```python
from build123d import *

# Parameters (mm, degrees)
SKETCH1_W            = 10
SKETCH1_H            = 80
BOSS_EXTRUDE1_DEPTH  = 51
SKETCH2_R            = 7.75
CUT_EXTRUDE1_DEPTH   = 45.1
SKETCH3_R            = 4.5
CUT_EXTRUDE2_DEPTH   = 96.399161422
SKETCH4_W            = 30
SKETCH4_H            = 80
SKETCH4_R            = 4.015
BOSS_EXTRUDE2_DEPTH  = 35
SKETCH4_3_R          = 4.015
BOSS_EXTRUDE3_DEPTH  = 30
CUT_EXTRUDE3_START   = -35
SKETCH5_W            = 24
SKETCH5_H            = 32
CUT_EXTRUDE3_DEPTH   = 35
SKETCH6_W            = 28
SKETCH6_H            = 32
CUT_EXTRUDE4_DEPTH   = 97.256168633
SKETCH12_W           = 10
SKETCH12_H           = 3
BOSS_EXTRUDE6_DEPTH  = 6
SKETCH14_R           = 1.6
CUT_EXTRUDE8_DEPTH   = 3
SKETCH14_2_R         = 1.6
CUT_EXTRUDE9_DEPTH   = 106.933941681
SKETCH15_R           = 4
CUT_EXTRUDE10_DEPTH  = 102.123686642
BOSS_EXTRUDE7_START  = 2.1
SKETCH16_R           = 7.5
SKETCH16_R_2         = 4
BOSS_EXTRUDE7_DEPTH  = 2.1
CUT_EXTRUDE11_START  = -14.5
SKETCH17_R           = 7.5
CUT_EXTRUDE11_DEPTH  = 14.5
SKETCH18_R           = 7.5
SKETCH18_R_2         = 4
BOSS_EXTRUDE8_DEPTH  = 5.45
SKETCH19_R           = 7
CUT_EXTRUDE12_DEPTH  = 17.8
SKETCH20_R           = 4
BOSS_EXTRUDE9_DEPTH  = 24
BOSS_EXTRUDE10_START = -24
SKETCH21_R           = 4
BOSS_EXTRUDE10_DEPTH = 24


with BuildPart() as part:
    # Sketch1 → Boss-Extrude1 (new body)
    with BuildSketch(Plane.XY):
        with Locations((5, 40)):
            Rectangle(SKETCH1_W, SKETCH1_H)
    extrude(amount=BOSS_EXTRUDE1_DEPTH)

    # Sketch2 → Cut-Extrude1 (cut)
    with BuildSketch(Plane.XY.offset(48)):
        with Locations((10, 9)):
            Circle(SKETCH2_R)
        with Locations((10, 71)):
            Circle(SKETCH2_R)
    extrude(amount=-CUT_EXTRUDE1_DEPTH, mode=Mode.SUBTRACT)

    # Sketch3 → Cut-Extrude2 (cut, through all)
    with BuildSketch(Plane.XY.offset(51)):
        with Locations((10, 71)):
            Circle(SKETCH3_R)
        with Locations((10, 9)):
            Circle(SKETCH3_R)
    extrude(amount=-CUT_EXTRUDE2_DEPTH, mode=Mode.SUBTRACT)

    # Sketch4 → Boss-Extrude2 (add)
    with BuildSketch(Plane.ZY):
        with Locations((25.5, 40)):
            Rectangle(SKETCH4_W, SKETCH4_H)
        with Locations((25.5, 71)):
            Circle(SKETCH4_R, mode=Mode.SUBTRACT)
        with Locations((25.5, 9)):
            Circle(SKETCH4_R, mode=Mode.SUBTRACT)
    extrude(amount=BOSS_EXTRUDE2_DEPTH)

    # Sketch4<3> → Boss-Extrude3 (add)
    with BuildSketch(Plane.ZY):
        with Locations((25.5, 71)):
            Circle(SKETCH4_3_R)
        with Locations((25.5, 9)):
            Circle(SKETCH4_3_R)
    extrude(amount=BOSS_EXTRUDE3_DEPTH)

    # Sketch5 → Cut-Extrude3 (cut)
    with BuildSketch(Plane.ZY.offset(35).offset(CUT_EXTRUDE3_START)):
        with Locations((25.5, 40)):
            Rectangle(SKETCH5_W, SKETCH5_H)
    extrude(amount=CUT_EXTRUDE3_DEPTH, mode=Mode.SUBTRACT)

    # Sketch6 → Cut-Extrude4 (cut, through all)
    with BuildSketch(Plane.XY.offset(40.5)):
        with Locations((-14, 40)):
            Rectangle(SKETCH6_W, SKETCH6_H)
    extrude(amount=-CUT_EXTRUDE4_DEPTH, mode=Mode.SUBTRACT)

    # Sketch12 → Boss-Extrude6 (add)
    with BuildSketch(Plane(origin=(0, 80, 0), x_dir=(1, 0, 0), z_dir=(0, 1, 0))):
        with Locations((5, -49.5)):
            Rectangle(SKETCH12_W, SKETCH12_H)
    extrude(amount=BOSS_EXTRUDE6_DEPTH)

    # Sketch14 → Cut-Extrude8 (cut)
    # profile 1 of 4: a face of its own
    with BuildSketch(Plane.ZY):
        Polygon((10.262029021, 55), (8.63101451, 57.825), (5.36898549, 57.825), (3.737970979, 55), (5.36898549, 52.175), (8.63101451, 52.175), align=None)
        with Locations((7, 55)):
            Circle(SKETCH14_R, mode=Mode.SUBTRACT)
    # profile 2 of 4: a face of its own
    with BuildSketch(Plane.ZY):
        Polygon((47.262029021, 55), (45.63101451, 57.825), (42.36898549, 57.825), (40.737970979, 55), (42.36898549, 52.175), (45.63101451, 52.175), align=None)
        with Locations((44, 55)):
            Circle(SKETCH14_R, mode=Mode.SUBTRACT)
    # profile 3 of 4: a face of its own
    with BuildSketch(Plane.ZY):
        Polygon((47.262029021, 25), (45.63101451, 27.825), (42.36898549, 27.825), (40.737970979, 25), (42.36898549, 22.175), (45.63101451, 22.175), align=None)
        with Locations((44, 25)):
            Circle(SKETCH14_R, mode=Mode.SUBTRACT)
    # profile 4 of 4: a face of its own
    with BuildSketch(Plane.ZY):
        Polygon((10.262029021, 25), (8.63101451, 27.825), (5.36898549, 27.825), (3.737970979, 25), (5.36898549, 22.175), (8.63101451, 22.175), align=None)
        with Locations((7, 25)):
            Circle(SKETCH14_R, mode=Mode.SUBTRACT)
    extrude(amount=-CUT_EXTRUDE8_DEPTH, mode=Mode.SUBTRACT)

    # Sketch14<2> → Cut-Extrude9 (cut, through all)
    with BuildSketch(Plane.ZY):
        with Locations((7, 55)):
            Circle(SKETCH14_2_R)
        with Locations((44, 55)):
            Circle(SKETCH14_2_R)
        with Locations((44, 25)):
            Circle(SKETCH14_2_R)
        with Locations((7, 25)):
            Circle(SKETCH14_2_R)
    extrude(amount=-CUT_EXTRUDE9_DEPTH, mode=Mode.SUBTRACT)

    # Sketch15 → Cut-Extrude10 (cut, through all)
    with BuildSketch(Plane(origin=(0, 80, 0), x_dir=(1, 0, 0), z_dir=(0, 1, 0))):
        with Locations(Location((-9, -18.3627, 0), (0, 0, 270))):
            Circle(SKETCH15_R)
        with Locations(Location((-22.925, -31.0373, 0), (0, 0, 270))):
            Circle(SKETCH15_R)
    extrude(amount=-CUT_EXTRUDE10_DEPTH, mode=Mode.SUBTRACT)

    # Sketch16 → Boss-Extrude7 (add)
    with BuildSketch(Plane(origin=(0, 24, 0), x_dir=(1, 0, 0), z_dir=(0, 1, 0)).offset(BOSS_EXTRUDE7_START)):
        with Locations(Location((-22.925, -31.0373, 0), (0, 0, 90))):
            Circle(SKETCH16_R)
        with Locations(Location((-22.925, -31.0373, 0), (0, 0, 270))):
            Circle(SKETCH16_R_2, mode=Mode.SUBTRACT)
    extrude(amount=-BOSS_EXTRUDE7_DEPTH)

    # Sketch17 → Cut-Extrude11 (cut)
    with BuildSketch(Plane.XZ.offset(CUT_EXTRUDE11_START)):
        with Locations(Location((-22.925, 31.0373, 0), (0, 0, 270))):
            Circle(SKETCH17_R)
    extrude(amount=CUT_EXTRUDE11_DEPTH, mode=Mode.SUBTRACT)

    # Sketch18 → Boss-Extrude8 (add)
    with BuildSketch(Plane.XZ.offset(-56)):
        with Locations(Location((-9, 18.3627, 0), (0, 0, 90))):
            Circle(SKETCH18_R)
        with Locations(Location((-9, 18.3627, 0), (0, 0, 90))):
            Circle(SKETCH18_R_2, mode=Mode.SUBTRACT)
    extrude(amount=BOSS_EXTRUDE8_DEPTH)

    # Sketch19 → Cut-Extrude12 (cut)
    with BuildSketch(Plane(origin=(0, 80, 0), x_dir=(1, 0, 0), z_dir=(0, 1, 0))):
        with Locations(Location((-9, -18.3627, 0), (0, 0, 270))):
            Circle(SKETCH19_R)
    extrude(amount=-CUT_EXTRUDE12_DEPTH, mode=Mode.SUBTRACT)

    # Sketch20 → Boss-Extrude9 (add)
    with BuildSketch(Plane(origin=(0, 24, 0), x_dir=(1, 0, 0), z_dir=(0, 1, 0))):
        with Locations(Location((-9, -18.3627, 0), (0, 0, 270))):
            Circle(SKETCH20_R)
    extrude(amount=-BOSS_EXTRUDE9_DEPTH)

    # Sketch21 → Boss-Extrude10 (add)
    with BuildSketch(Plane.XZ.offset(-56).offset(BOSS_EXTRUDE10_START)):
        with Locations(Location((-22.925, 31.0373, 0), (0, 0, 90))):
            Circle(SKETCH21_R)
    extrude(amount=BOSS_EXTRUDE10_DEPTH)


solid = part.part
```
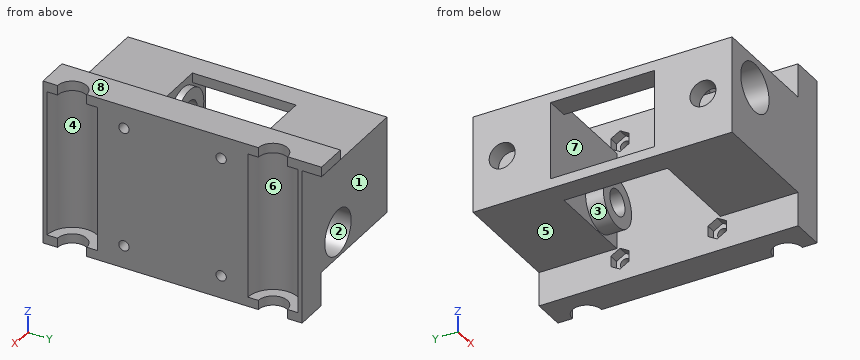
Build history of the part. All positions in model axes, mm. Face numbers are marked on the shaded views. A direction names the side the tool comes from. Round coordinates to 2 decimals unless told otherwise and drop trailing zeros. Write each loop counter-clockwise with the first axis right and the second up, starting at its lowest first coordinate (ties: lowest second). Pieces come first, ordered by that corner, then holes.
1) Band-saw the part on A-A, the plane z = 7. List the corners of the cut face in (x, y) (3 decimals).
2) Drill centre lines: probe 1 along Y at (x, z) = (1, 44) (3 decimals); probe 2 along Y at (x, z) = (-24.5, 25.5); probe 3 along X at (y, z) = (34, 40). Where is each one in solid material? Low to high.
3) 3-axis set-ups, long thin cutter, end or side, ignore diameter. For the marked faces 1, 2, 3, 4 and 5: which of +Z, -Z, +X, -X, +Y, -Y reach the whole face in a straight line?
4) Band-saw the part on C-C, the plane y = 43. List the corners of the cut face in (x, z), and give its area (3 significant figures).
5) Band-saw the part on D-D, the plane z = 16. List the corners of the cut face in (x, y), and give its area (3 significant figures).
6) Mould opens along X. For the marked faces 6, 7 and 8 say: +X half, -X half, draft (parallel to the pull), parting line (faces both ways), or undercut.
7) Pin check, flat tips, straight feed: pin 1 (1 mm diameter, centred on x = -20.5, y = 11.5, fed in from -Z); pin 2 (9 mm diameter, centred on x = -19.5, z = 30, fed in from +Y); pin 3 (1.7 mm diameter, centred on y = 26.5, z = 44.5, fed in from -X). Stop position of each tip, or through.
8) Band-saw the part on B-B, the plane x = -9. List the corners of the cut face in (y, z), and give its area (3 significant figures).
Ans:
1. outline: (0, 0) - (10, 0) - (10, 1.25) arc R7.75 cw to (10, 16.75) - (10, 23.4) - (3, 23.4) - (3, 22.175) - (0, 22.175) - close; (0, 27.825) - (3, 27.825) - (3, 26.6) - (10, 26.6) - (10, 53.4) - (3, 53.4) - (3, 52.175) - (0, 52.175) - close; (0, 57.825) - (3, 57.825) - (3, 56.6) - (10, 56.6) - (10, 63.25) arc R7.75 cw to (10, 78.75) - (10, 80) - (0, 80) - close
2. probe 1: y = 0 to 22.175, 27.825 to 52.175, 57.825 to 80
2. probe 2: y = 14.5 to 26.1, 56 to 80
2. probe 3: x = -35 to -28, 0 to 10
3. face 1: -Z, +X, -X, +Y
3. face 2: +Y
3. face 3: none
3. face 4: +X
3. face 5: -Z, -X, +Y, -Y
4. outline: (-35, 10.5) - (-28, 10.5) - (-28, 13.5) - (-35, 13.5) - close; (-35, 37.5) - (-28, 37.5) - (-28, 40.5) - (-35, 40.5) - close; (0, 0) - (10, 0) - (10, 51) - (0, 51) - close
4. area: 552 mm2
5. outline: (-35, 0) - (10, 0) - (10, 1.25) arc R7.75 cw to (10, 16.75) - (10, 63.25) arc R7.75 cw to (10, 78.75) - (10, 80) - (-2.41, 80) - (-2.41, 62.2) - (-5.77, 62.2) - (-5.77, 50.55) - (-1.88, 50.55) - (-1.88, 56) - (0, 56) - (0, 24) - (-35, 24) - close; (-35, 56) - (-16.12, 56) - (-16.12, 50.55) - (-12.23, 50.55) - (-12.23, 62.2) - (-15.59, 62.2) - (-15.59, 80) - (-35, 80) - close
5. area: 2,060 mm2
6. face 6: +X half
6. face 7: undercut
6. face 8: draft
7. pin 1: stops at z = 10.5
7. pin 2: stops at y = 80
7. pin 3: stops at x = 3
8. outline: (0, 10.5) - (24, 10.5) - (24, 40.5) - (0, 40.5) - close; (50.55, 10.86) - (56, 10.86) - (56, 10.5) - (80, 10.5) - (80, 11.36) - (62.2, 11.36) - (62.2, 14.36) - (50.55, 14.36) - close; (50.55, 22.36) - (62.2, 22.36) - (62.2, 25.36) - (80, 25.36) - (80, 40.5) - (56, 40.5) - (56, 25.86) - (50.55, 25.86) - close
8. area: 1,180 mm2
